The figure shows three views and two pictorial views of one solid part (mm, origin at its lowest corner). Answer the questions. A direction names the side the tool comes from. Coordinates: 2 decimals unless noted, no trailing zeros. Loops run counter-clockwise (first coordinate to the right, second up) from the corner with the lowest first, then second, coordinate; pieces in that order, holes last. Notation, with made-up numbers: M -25,4.25 L -5,4.25 A22 cw -5,31.25 Z; hole C 44.5,7.5 d5. An arc over 180 degrees is marked long. One line per item, written item: value. Start each with the question number.
1. The part is cut by section B-B (y = 7.62). Write down the section's boundary in (x, z), then the cut area to 3 significant figures.
2. The part is cut by section C-C (z = 17). Write down the section's boundary in (x, y).
3. The part is cut by section A-A (x = 24.13). Write down the section's boundary in (y, z), then the cut area to 3 significant figures.
4. Determine the mould class of the marked faces 4, 5 and 6 for opening direction X: +X half, -X half, draft (parallel to the pull), parting line (faces both ways), or undercut.
5. The part is cut by section D-D (y = 31). Write down the section's boundary in (x, z).
6. Consider probe 1 along X at (y, z) = (15.24, 2.75) (1 decimal); probe 2 along X at (y, z) = (7.62, 6.5); probe 3 along Y at (x, z) = (25.5, 21.5). Determine where each line is inside the solid, lowest interval first.
7. For the marked faces 1, 2 and 3, determine the directions among +Z, -Z, +X, -X, +Y, -Y from which every point of the face is accessible in a straight line to the end or side of a thin tool.
8. Flat-ended cylindrical pins translate along their axes: pin 1 (14 mm diameter, centred on x = 25, z = 23, fed in from -Y); pin 2 (10 mm diameter, centred on x = 5, y = 25, fed in from +Z); pin 3 (5 mm diameter, centred on y = 55.5, z = 23.5, fed in from -X). Find the tip coordinate at first contact, or state that the pin passes through.
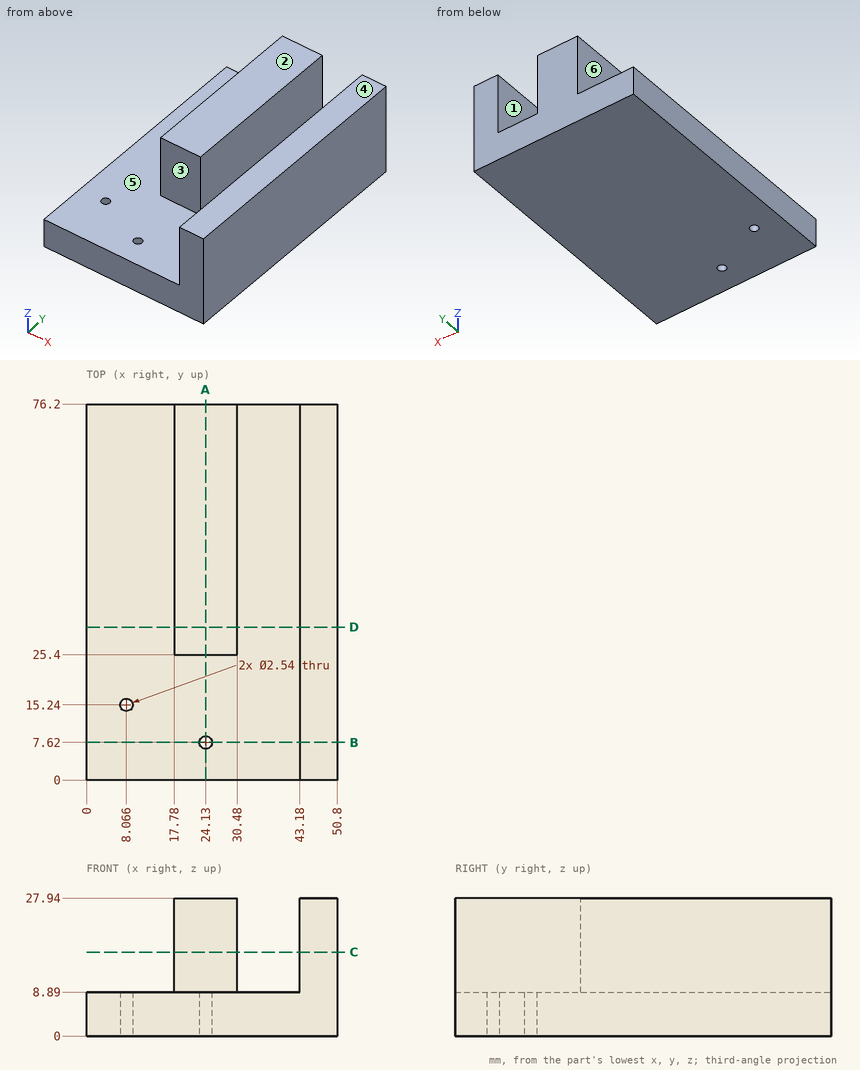
Answer block:
1. outline: M 0,0 L 22.86,0 L 22.86,8.89 L 0,8.89 Z; M 25.4,0 L 50.8,0 L 50.8,27.94 L 43.18,27.94 L 43.18,8.89 L 25.4,8.89 Z
1. area: 574 mm2
2. outline: M 17.78,25.4 L 30.48,25.4 L 30.48,76.2 L 17.78,76.2 Z; M 43.18,0 L 50.8,0 L 50.8,76.2 L 43.18,76.2 Z
3. outline: M 0,0 L 6.35,0 L 6.35,8.89 L 0,8.89 Z; M 8.89,0 L 76.2,0 L 76.2,27.94 L 25.4,27.94 L 25.4,8.89 L 8.89,8.89 Z
3. area: 1,620 mm2
4. face 4: draft
4. face 5: undercut
4. face 6: -X half
5. outline: M 0,0 L 50.8,0 L 50.8,27.94 L 43.18,27.94 L 43.18,8.89 L 30.48,8.89 L 30.48,27.94 L 17.78,27.94 L 17.78,8.89 L 0,8.89 Z
6. probe 1: x = 0 to 6.8, 9.3 to 50.8
6. probe 2: x = 0 to 22.86, 25.4 to 50.8
6. probe 3: y = 25.4 to 76.2
7. face 1: +Z, +Y, -Y
7. face 2: +Z, +X, -X, +Y, -Y
7. face 3: +Z, -X, -Y
8. pin 1: stops at y = 25.4
8. pin 2: stops at z = 8.89
8. pin 3: stops at x = 17.78
